```python
from build123d import *

# Parameters (mm, degrees)
F1_DEPTH = 2.5
F2_R     = 0.5
F3_R     = 0.5


with BuildPart() as f1:
    # F0 (on Top) → F1 (new body)
    with BuildSketch(Plane.XY):
        Polygon((-20.4225578644, -6.6356912976), (-12.6218348974, 17.372465356), (-53.4669506262, 17.372465356), align=None)
        Polygon((12.6218348974, 17.372465356), (0, 56.2184788287), (-12.6218348974, 17.372465356), align=None)
        Polygon((12.6218348974, 17.372465356), (-12.6218348974, 17.372465356), (-20.4225578644, -6.6356912976), (0, -21.4735481167), (20.4225578644, -6.6356912976), align=None)
        Polygon((53.4669506262, 17.372465356), (12.6218348974, 17.372465356), (20.4225578644, -6.6356912976), align=None)
        Polygon((33.0443927618, -45.4817047703), (20.4225578644, -6.6356912976), (0, -21.4735481167), align=None)
        Polygon((0, -21.4735481167), (-20.4225578644, -6.6356912976), (-33.0443927618, -45.4817047703), align=None)
    extrude(amount=F1_DEPTH)

    # F2
    f2_edges = [f1.edges().sort_by_distance(p)[0] for p in [
        (0, 56.218479, 1.25),
        (-53.466951, 17.372465, 1.25),
        (-33.044393, -45.481705, 1.25),
        (33.044393, -45.481705, 1.25),
        (53.466951, 17.372465, 1.25),
        (-20.422558, -6.635691, 1.25),
        (-12.621835, 17.372465, 1.25),
        (12.621835, 17.372465, 1.25),
        (20.422558, -6.635691, 1.25),
        (0, -21.473548, 1.25),
    ]]
    fillet(f2_edges, radius=F2_R)

    # F3
    f3_edges = [f1.edges().sort_by_distance(p)[0] for p in [
        (6.492553, 36.236455, 2.5),
        (-6.492553, 36.236455, 2.5),
        (32.456608, 17.372465, 2.5),
        (36.469226, 5.022896, 2.5),
        (26.55184, -25.499681, 2.5),
        (16.046668, -33.132135, 2.5),
        (-16.046668, -33.132135, 2.5),
        (-26.55184, -25.499681, 2.5),
        (-36.469226, 5.022896, 2.5),
        (-32.456608, 17.372465, 2.5),
        (-32.387229, -44.577196, 2.5),
        (32.387229, -44.577196, 2.5),
        (52.403637, 17.026974, 2.5),
        (0, 55.100445, 2.5),
        (-52.403637, 17.026974, 2.5),
    ]]
    fillet(f3_edges, radius=F3_R)


solid = f1.part
```
Check sheet for the modelled part. Datum: model origin and axes. Units: mm. A direction names the side the tool comes from. Round coordinates to 2 decimals unless told otherwise and drop trailing zeros. Order: outer loops, then holes, each group sorted by start corner. A loop starts at its lowest first (then second) coordinate and runs counter-clockwise, first axis right, second up.
1) Go/stop test with flat-tipped pins: pin 1 Ø1 at (x, z) = (25, 0.5) entering from +Y; pin 2 Ø1 at (x, y) = (13, 2.5) entering from -Z; pin 3 Ø1 at (x, z) = (27.5, 2) entering from -Y. Record where each tip stops, or that it passes through.
2) Mould release check, pull along Y, two halves, no side actions. Record for faces 6 (the cylindrical face through (16.36, -33.17, 2.36)), 7 (the flat face through (36.249, 4.863, 0.986)), 8 (the cylindrical face through (6.265, 36.449, 2.357)): +Y half, -Y half, draft (parallel to the pull), parting line (faces both ways), or undercut.
3) Scan lines: line 1 (X direction, y = -23, z = 2); line 2 (X direction, y = 18, z = 0.6); line 3 (X direction, y = -22.5, z = 1.95). Record each from-to range of solid material in increasing order.
4) Tool access check on faces 1 (the cylindrical face through (26.32, -25.29, 2.36)), 2 (the flat face through (26.636, -25.759, 0.986)), 3 (the flat face through (15.826, -32.972, 0.986)), 4 (the flat face through (-36.69, 5.183, 0.986)), 5 (the cylindrical face through (-36.16, 4.984, 2.357)). Record the directions out of +Z, -Z, +X, -X, +Y, -Y that give a thin tool (end or side, any length) a straight path to the whole face; none if there is none.
5) Section check A-A (z = 1.1). Record the boundary of the cut face in (x, y), and give its area (3 significant figures).
Result:
1. pin 1: stops at y = 17.37
1. pin 2: stops at z = 0
1. pin 3: stops at y = -41.82
2. face 6: -Y half
2. face 7: undercut
2. face 8: +Y half
3. line 1: x = -25.74 to -2.1, 2.1 to 25.74
3. line 2: x = -12.42 to 12.42
3. line 3: x = -25.58 to -1.41, 1.41 to 25.58
4. face 1: +Z, +X
4. face 2: +Z, -Z, +X
4. face 3: +Z, -Z, -Y
4. face 4: +Z, -Z, -X
4. face 5: +Z, -X
5. outline: (-52.22, 16.47) - (-20.72, -6.42) arc R0.5 cw to (-20.53, -6.98) - (-32.57, -44.02) arc R0.5 ccw to (-31.8, -44.58) - (-0.29, -21.69) arc R0.5 cw to (0.29, -21.69) - (31.8, -44.58) arc R0.5 ccw to (32.57, -44.02) - (20.53, -6.98) arc R0.5 cw to (20.72, -6.42) - (52.22, 16.47) arc R0.5 ccw to (51.93, 17.37) - (12.99, 17.37) arc R0.5 cw to (12.51, 17.72) - (0.48, 54.75) arc R0.5 ccw to (-0.48, 54.75) - (-12.51, 17.72) arc R0.5 cw to (-12.99, 17.37) - (-51.93, 17.37) arc R0.5 ccw to start
5. area: 3,550 mm2
